Could you check a few things on this drawing? It's one solid part, dimensions in mm from its lowest x, y, z. A direction names the side the tool comes from. Coordinates: 2 decimals unless noted, no trailing zeros. Write each loop counter-clockwise with the first axis right and the second up, starting at its lowest first coordinate (ties: lowest second). Pieces come first, ordered by that corner, then holes.
Item 1: For the marked faces 1 and 2, which set-ups out of +Z, -Z, +X, -X, +Y, -Y let a thin tool reach every point of the face, with its end or its side?
Item 2: Please list where these lines run through material, in increasing order: line 1 (X direction, y = 16.5, z = 30.5) (1 decimal); line 2 (Z direction, x = 66, y = 17.55); line 3 (Z direction, x = 60, y = 14.5).
Item 3: I'm going to push flat-ended pins straight in: P1, Ø1.8, axis at x = 65.5, z = 28.5, coming from the +Y side; P2, Ø1.5, axis at y = 11, z = 8, coming from the -X side; P3, Ø1.5, axis at x = 13.5, z = 52, coming from the +Y side. Where does each tip first touch, or does it pass through?
Item 4: I want a section at A-A (y = 15.25). Please give me the cut outline in (x, z).
Item 5: If we mould it in two halves opening along Z, with no side actions, what happens to the marked faces 3, 4 and 5? For each: pulls with the +Z half, pulls with the -Z half, needs draft (parallel to the pull), parting line crosses it, or undercut.
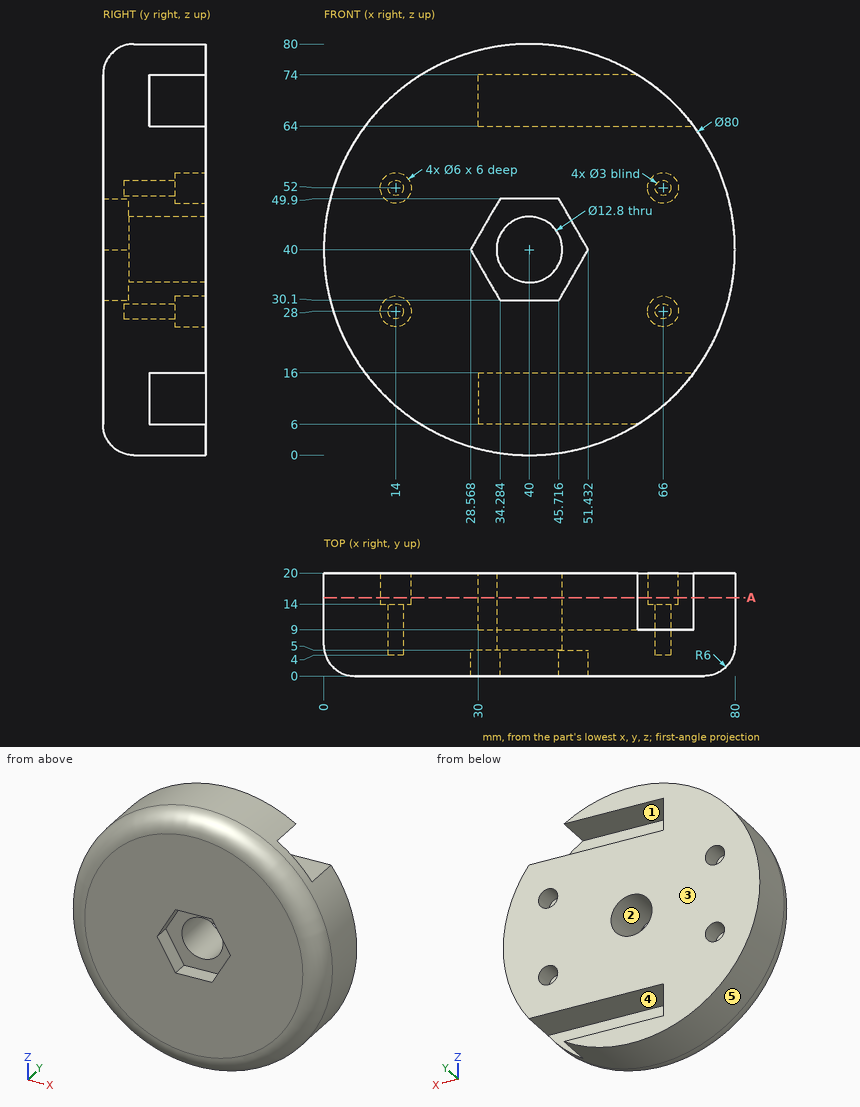
Answer:
1. face 1: +X, +Y
1. face 2: +Y, -Y
2. line 1: x = 1.1 to 12.3, 15.7 to 64.3, 67.7 to 78.9
2. line 2: z = 16 to 25, 31 to 49, 55 to 64
2. line 3: z = 5.36 to 6, 16 to 64, 74 to 74.64
3. P1: stops at y = 14
3. P2: stops at x = 15.03
3. P3: stops at y = 4
4. outline: (30, 6) - (30, 16) - (72, 16) arc R40 ccw to (72, 64) - (30, 64) - (30, 74) - (61.07, 74) arc R40 ccw (long way) to (61.07, 6) - close; hole circle Ø6 at (14, 28); hole circle Ø6 at (14, 52); hole circle Ø12.8 at (40, 40); hole circle Ø6 at (66, 28); hole circle Ø6 at (66, 52)
5. face 3: needs draft
5. face 4: undercut
5. face 5: parting line crosses it
